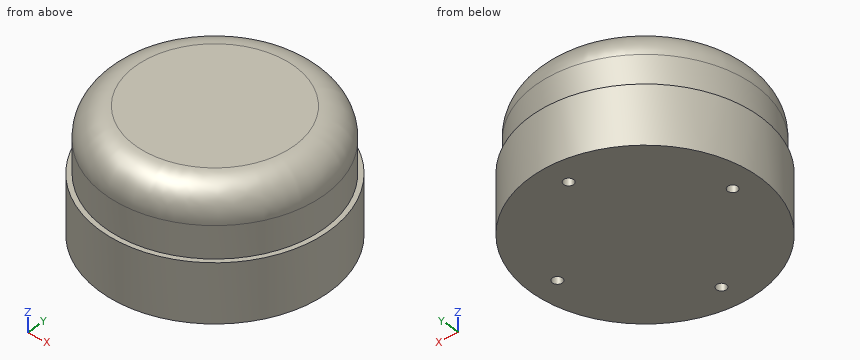
```python
from build123d import *

# Parameters (mm, degrees)
F0_R     = 37.85
F1_DEPTH = 19.4
F3_D     = 3.3
F3_DEPTH = 4
F3_TIP   = 0.9914200214


with BuildPart() as f1:
    # F0 (on Top) → F1 (new body)
    with BuildSketch(Plane.XY):
        Circle(F0_R)
    extrude(amount=F1_DEPTH)

    # F3
    with Locations(Plane(origin=(0, 0, 0), x_dir=(1, 0, 0), z_dir=(0, 0, -1))):
        with Locations((0, 29.5), (-29.5, 0), (0, -29.5), (29.5, 0)):
            Hole(F3_D / 2, depth=F3_DEPTH)
            with Locations((0, 0, -(F3_DEPTH + F3_TIP / 2))):  # 118° drill point
                Cone(0, F3_D / 2, F3_TIP, mode=Mode.SUBTRACT)

    # F4 (on Right) → F5 (revolve)
    with BuildSketch(Plane.YZ):
        with BuildLine():
            Line((-36.25, 29.9819558859), (-36.25, 19.4))
            Line((-36.25, 19.4), (0, 19.4))
            Line((0, 19.4), (0, 40.8))
            Line((0, 40.8), (-26.2835159747, 40.8))
            ThreePointArc((-26.2835159747, 40.8), (-33.6381213734, 37.57567557), (-36.25, 29.9819558859))
        make_face()
    revolve(axis=Axis((0, 0, 30.1), (0, 0, 1)))


solid = f1.part
```
CAD build for the part. Positions are in the model's coordinates, mm. Round coordinates to 2 decimals unless told otherwise and drop trailing zeros. Write each loop counter-clockwise with the first axis right and the second up, starting at its lowest first coordinate (ties: lowest second). Pieces come first, ordered by that corner, then holes. Notation, with made-up numbers: (56.25, 30.25) - (104.25, 30.25) arc R21 ccw to (104.25, 68.25) - close; hole circle Ø3 at (-27.75, 9.25). An arc over 180 degrees is marked (long way). Return JSON: item names as keys, results as strings. Group by question number.
Item 1: Probe probe 1 along Y at (x, z) = (0, 0.85); probe 2 along X at (y, z) = (-29.5, 2.85); probe 3 along Y at (x, z) = (29, 2). List the from-to ranges inside material, lowest first.
Item 2: Flat gauge pins, fed straight in: pin 1 Ø6 at (x, z) = (18, 32) entering from +Y; pin 2 Ø1 at (x, z) = (-10, 14.5) entering from -Y; pin 3 Ø10 at (x, z) = (6, 11) entering from -Y; pin 4 Ø12 at (x, y) = (25.5, -18.5) entering from +Z. Where does each tip first touch, or does it go through?
Item 3: Band-saw the part on A-A on z = 11. List the corners of the cut face in (x, y).
Resolved:
{
 "1": {"probe 1": "y = -37.85 to -31.15, -27.85 to 27.85, 31.15 to 37.85", "probe 2": "x = -23.71 to -1.65, 1.65 to 23.71", "probe 3": "y = -24.32 to -1.57, 1.57 to 24.32"},
 "2": {"pin 1": "stops at y = 32.99", "pin 2": "stops at y = -36.64", "pin 3": "stops at y = -37.84", "pin 4": "stops at z = 40.8"},
 "3": {"outline": "circle Ø75.7 at (0, 0)"}
}
